Can you work these out from the model? Positions are in its coordinate system, mm. A direction names the side the tool comes from. Give positions to 0.01 mm unless a question says otherwise; leave off trailing zeros. Order: outer loops, then holes, each group sorted by start corner. A loop starts at its lowest first (then second) coordinate and runs counter-clockwise, first axis right, second up. Notation, with made-up numbers: (-14.5, -7) -> (6.5, -7) arc R22 ccw to (6.5, 3) -> close; hole circle Ø2 at (-24.5, -18). An arc over 180 degrees is marked (long way). Answer as a JSON object with one key per item and string values.
Autodesk Inventor part; units mm, degrees
ref_plane "YZ Plane" through (0, 0, 0) normal (1, 0, 0) x (0, 1, 0)
ref_plane "XZ Plane" through (0, 0, 0) normal (0, 1, 0) x (-1, 0, 0)
ref_plane "XY Plane" through (0, 0, 0) normal (0, 0, 1) x (1, 0, 0)
sketch "Sketch1" plane through (0, 0, 0) normal (0, 0, 1) x (1, 0, 0)
  line L0 (0, 0) -> (133.35, 0)
  line L1 (133.35, 0) -> (133.35, 50.8)
  line L2 (0, 50.8) -> (0, 0)
  line L3 (0, 50.8) -> (6.35, 50.8)
  line L4 (6.35, 50.8) -> (6.35, 6.35)
  line L5 (6.35, 6.35) -> (127, 6.35)
  line L6 (127, 6.35) -> (127, 50.8)
  line L7 (127, 50.8) -> (133.35, 50.8)
  dimension "d1" = 50.8
  dimension "d2" = 6.35
  dimension "d3" = 44.45
  dimension "d4" = 120.65
  dimension "d5" = 133.35
extrude "Extrusion1" add sketch "Sketch1" along normal blind 6.35
fillet "Fillet1" radius 3.175 2 edges at (66.675, 0, 6.35) (66.675, 0, 0)
sketch "Sketch2" plane through (0, 50.8, 0) normal (0, 1, 0) x (1, 0, 0)
  line L0 (6.35, -6.35) -> (16.515747, 6.26204)
  line L1 (-2.903527, -17.830303) -> (6.35, -6.35)
  line L2 (16.515747, 6.26204) -> (9.563953, 11.86543)
  line L3 (9.563953, 11.86543) -> (-9.855321, -12.226913)
  line L4 (-9.855321, -12.226913) -> (-2.903527, -17.830303)
  line L5 (127, 0) -> (127, -6.35)
  line L6 (127, -6.35) -> (143.198942, -6.35) construction
  line L7 (116.834265, 6.26204) -> (123.786067, 11.86543)
  line L8 (123.786067, 11.86543) -> (143.205318, -12.226913)
  line L9 (143.205318, -12.226913) -> (136.253516, -17.830303)
  line L10 (133.35, -6.35) -> (127, -6.35)
  line L11 (116.834265, 6.26204) -> (136.253516, -17.830303)
  point P0 (0, 0)
extrude "Extrusion2" add sketch "Sketch2" along normal blind 6.35
sketch "Sketch6" plane through (16.515747, 50.8, -6.26204) normal (0.7785715, 0, 0.6275559) x (0.6275559, 0, -0.7785715)
  line L0 (-30.944292, 6.35) -> (0, 6.35)
  line L1 (-30.944292, 0) -> (-30.944292, 6.35)
  line L2 (-30.944292, 6.35) -> (-30.944292, 0)
  line L3 (0, 0) -> (0, 6.35)
  line L4 (-30.944292, 0) -> (0, 0)
  line L5 (0, 0) -> (0, 6.35)
  line L6 (0, 6.35) -> (-30.944292, 6.35)
  point P0 (-15.240001, -50.8)
extrude "Extrusion3" add sketch "Sketch6" along normal blind 1.5875
sketch "Sketch7" plane through (-9.855321, 50.8, 12.226913) normal (-0.7785715, 0, -0.6275559) x (-0.6275559, 0, 0.7785715)
  line L0 (-30.944292, 6.35) -> (0, 6.35)
  line L1 (0, 0) -> (-30.944292, 0)
  line L2 (-30.944292, 6.35) -> (-30.944292, 0)
  line L3 (-30.944292, 0) -> (0, 0)
  line L4 (0, 6.35) -> (0, 0)
  line L5 (0, 0) -> (0, 6.35)
  line L6 (0, 6.35) -> (-30.944292, 6.35)
  point P0 (-15.704291, -50.8)
extrude "Extrusion4" add sketch "Sketch7" along normal blind 1.5875
sketch "Sketch8" plane through (136.253516, 50.8, 17.830303) normal (-0.7785718, 0, 0.6275555) x (0.6275555, 0, 0.7785718)
  line L0 (-30.944277, 6.35) -> (0, 6.35)
  line L1 (0, 0) -> (0, 6.35)
  line L2 (-30.944277, 6.35) -> (0, 6.35)
  line L3 (0, 6.35) -> (0, 0)
  line L4 (0, 0) -> (-30.944277, 0)
  line L5 (-30.944277, 0) -> (-30.944277, 6.35)
  line L6 (-30.944277, 0) -> (-30.944277, 6.35)
  point P0 (-99.388813, -50.8)
extrude "Extrusion5" add sketch "Sketch8" along normal blind 1.5875
sketch "Sketch9" plane through (123.786067, 50.8, -11.86543) normal (0.7785718, 0, -0.6275555) x (-0.6275555, 0, -0.7785718)
  line L0 (-30.944277, 6.35) -> (0, 6.35)
  line L1 (-30.944277, 6.35) -> (0, 6.35)
  line L2 (0, 0) -> (-30.944277, 0)
  line L3 (0, 6.35) -> (0, 0)
  line L4 (0, 0) -> (-30.944277, 0)
  line L5 (-30.944277, 0) -> (-30.944277, 6.35)
  point P0 (68.444536, -50.8)
extrude "Extrusion6" add sketch "Sketch9" along normal blind 1.5875
fillet "Fillet4" radius 6.35 8 edges at (133.35, 50.8, 3.175) (130.175, 50.8, 0) (127, 50.8, 3.175) (130.175, 50.8, 6.35) (6.35, 50.8, 3.175) (3.175, 50.8, 6.35) (0, 50.8, 3.175) (3.175, 50.8, 0)
properties part number "landing_3DPrint"
1. If we section it at A-A on y = 29: Please give me the cut outline in (x, z).
Worked answers:
{"outline": "(0, 0) -> (6.35, 0) -> (6.35, 6.35) -> (0, 6.35) -> close; (127, 0) -> (133.35, 0) -> (133.35, 6.35) -> (127, 6.35) -> close"}
2. If we section it at B-B on z = 16.5: Please give me the cut outline in (x, y), then the cut area to 3 significant figures.
Worked answers:
{"outline": "(-4.55, 50.8) -> (0.21, 50.8) -> (0.21, 57.15) -> (-4.55, 57.15) -> close; (133.14, 50.8) -> (137.9, 50.8) -> (137.9, 57.15) -> (133.14, 57.15) -> close", "area": "60.5 mm²"}
3. For faces 1 (the face through (66, 6, 6.35)), 2 (the face through (6.35, 26, 3)), 3 (the face through (120.244, 54.019, -9.011)), 4 (the face through (0, 23, 3)), 5 (the face through (125.17, 53.68, 6.61)), which set-ups out of +Z, -Z, +X, -X, +Y, -Y let a thin tool reach every point of the face, with its end or its side?
Worked answers:
{"face 1": "+Z, +X, -X, -Y", "face 2": "+Z, -Z", "face 3": "-Z, +Y, -Y", "face 4": "+Z, -Z, -X, -Y", "face 5": "+Z, +Y"}
4. Please list where these lines run through material, in increasing order: L1, parallel to X at y = 21, z = 1; L2, parallel to Z at x = 1, y = 21.5.
Worked answers:
{"L1": "0 to 6.35, 127 to 133.35", "L2": "0 to 6.35"}
5. Will these pins go through, and if not, where does the flat tip stop? pin 1 Ø1.9 at (y, z) = (20, 5) entering from +X; pin 2 Ø5 at (y, z) = (18, 3) entering from -X; pin 3 Ø6 at (x, y) = (9.5, 32) entering from -Z; pin 4 Ø8 at (x, y) = (5.5, 34.5) entering from -Z.
Worked answers:
{"pin 1": "x = 133.35", "pin 2": "x = 0", "pin 3": "through", "pin 4": "z = 0"}
6. If we mould it in two halves opening along Y, with no side actions, what happens to faces 6 (the face through (139.663, 53.931, 15.082)), 7 (the face through (-1.91, 48.99, 4.15)), 8 (the face through (125.09, 48.99, 2))? For each: +Y half, -Y half, draft (parallel to the pull), parting line (faces both ways), or undercut.
Worked answers:
{"face 6": "draft", "face 7": "-Y half", "face 8": "undercut"}
